Check sheet for the drawn part. Datum: minimum x, y, z corner. Units: mm. A direction names the side the tool comes from. Round coordinates to 2 decimals unless told otherwise and drop trailing zeros. Write each loop counter-clockwise with the first axis right and the second up, starting at its lowest first coordinate (ties: lowest second). Pieces come first, ordered by that corner, then holes. Notation, with made-up numbers: M 36,2.5 L 53,2.5 A23 cw 53,24.5 Z; hole C 27,89 d6. An arc over 180 degrees is marked long. Answer in a Markdown table with one row per item. Add a question column.
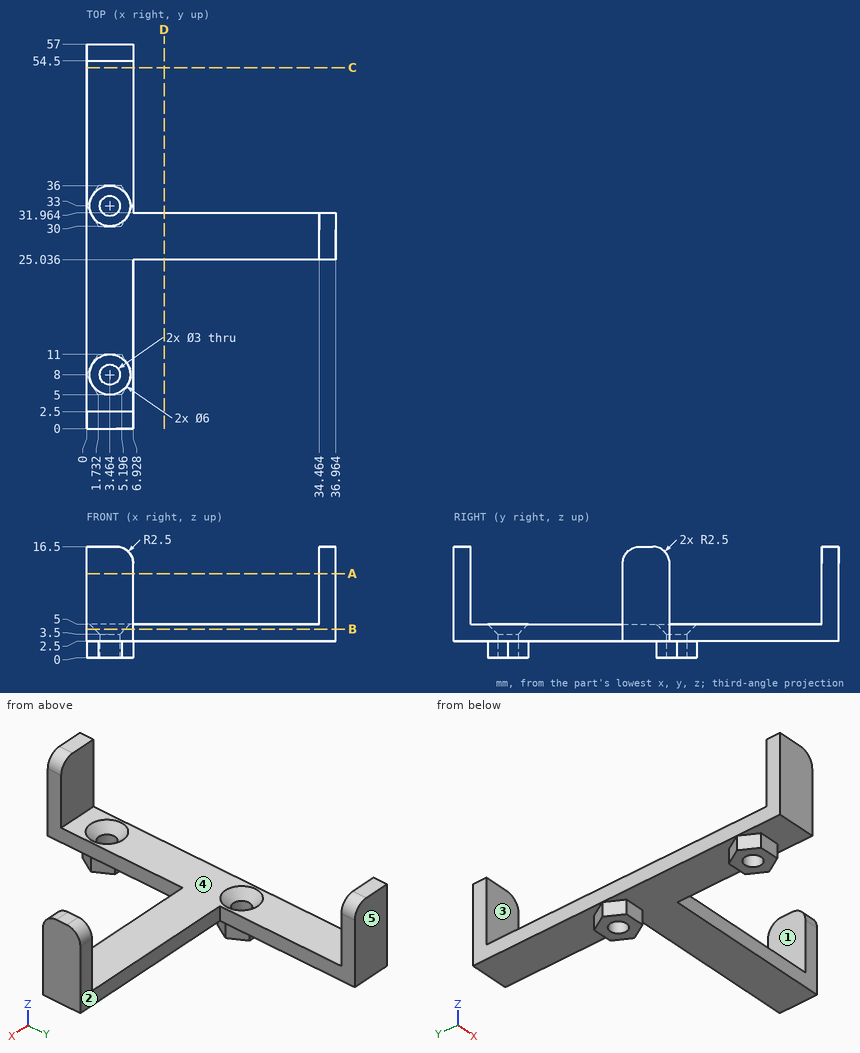
Item 1: Access from +Z, -Z, +X, -X, +Y, -Y to the whole of each face (thin tool, end or side, straight path). Record for the marked faces 1, 2, 3, 4 and 5.
Item 2: Gauge pin test, flat ends, axial feed: pin 1 Ø5.5 at (x, y) = (2, 45) entering from -Z; pin 2 Ø1.2 at (x, z) = (4, 1) entering from -Y; pin 3 Ø6 at (x, y) = (27, 36.5) entering from -Z (3 decimals); pin 4 Ø7.5 at (y, z) = (29.5, 13.5) entering from -X. Record the tip position at first contact, or that the pin passes through.
Item 3: Section check B-B, the plane z = 4.25. Record the boundary of the cut face in (x, y), and give its area (3 significant figures).
Item 4: Scan lines: probe 1 along Y at (x, z) = (5, 10.25); probe 2 along X at (y, z) = (8, 2.2); probe 3 along Y at (x, z) = (8.5, 3.5). Record each from-to range of solid material in increasing order. Write a range as from..to.
Item 5: Section check A-A, the plane z = 12.5. Record the boundary of the cut face in (x, y).
Item 6: Section check D-D, the plane x = 11.5. Record the boundary of the cut face in (y, z).
Item 7: Section check C-C, the plane y = 53.5. Record the boundary of the cut face in (x, z), and give its area (3 significant figures).
Result sheet:
| question | item | result |
|---|---|---|
| 1 | face 1 | +Z, -X, +Y, -Y |
| 1 | face 2 | +Z, -Z, +X, +Y |
| 1 | face 3 | +Z, +X, -X |
| 1 | face 4 | +Z, -X |
| 1 | face 5 | +Z, -Z, +X, -X, +Y |
| 2 | pin 1 | stops at z = 2.5 |
| 2 | pin 2 | stops at y = 5 |
| 2 | pin 3 | passes through |
| 2 | pin 4 | stops at x = 34.46 |
| 3 | outline | M 0,0 L 6.93,0 L 6.93,25.04 L 36.96,25.04 L 36.96,31.96 L 6.93,31.96 L 6.93,57 L 0,57 Z; hole C 3.46,8 d4.5; hole C 3.46,33 d4.5 |
| 3 | area | 571 mm^2 |
| 4 | probe 1 | y = 0..2.5, 54.5..57 |
| 4 | probe 2 | x = 0..1.96, 4.96..6.93 |
| 4 | probe 3 | y = 25.04..31.96 |
| 5 | outline | M 0,0 L 6.93,0 L 6.93,2.5 L 0,2.5 Z; M 0,54.5 L 6.93,54.5 L 6.93,57 L 0,57 Z; M 34.46,25.04 L 36.96,25.04 L 36.96,31.96 L 34.46,31.96 Z |
| 6 | outline | M 25.04,2.5 L 31.96,2.5 L 31.96,5 L 25.04,5 Z |
| 7 | outline | M 0,2.5 L 6.93,2.5 L 6.93,5 L 0,5 Z |
| 7 | area | 17.3 mm^2 |
